```python
from build123d import *

# Parameters (mm, degrees)
CUT_EXTRUDE1_START = -20
CUT_EXTRUDE1_DEPTH = 20


with BuildPart() as part:
    # Sketch1 → Revolve1 (revolve)
    with BuildSketch(Plane.XY, mode=Mode.PRIVATE) as revolve1_sk:
        Polygon((0, 22.5), (4, 22.5), (4, -4), (10, -4), (10, -6), (0, -6), align=None)
    revolve(revolve1_sk.sketch.rotate(Axis((0, -6, 0), (0, 1, 0)), 90), axis=Axis((0, -6, 0), (0, 1, 0)))

    # Sketch2 → Cut-Extrude1 (cut)
    with BuildSketch(Plane(origin=(0, 22.5, 0), x_dir=(1, 0, 0), z_dir=(0, 1, 0)).offset(CUT_EXTRUDE1_START)):
        with BuildLine():
            Line((-2.645751311, -3), (2.645751311, -3))
            ThreePointArc((2.645751311, -3), (0, -4), (-2.645751311, -3))
        make_face()
    extrude(amount=CUT_EXTRUDE1_DEPTH, mode=Mode.SUBTRACT)


solid = part.part
```
Input: part model. Units: mm. Frame: model coordinates. A direction names the side the tool comes from. Give positions to 0.01 mm unless a question says otherwise; leave off trailing zeros. Write each loop counter-clockwise with the first axis right and the second up, starting at its lowest first coordinate (ties: lowest second). Pieces come first, ordered by that corner, then holes. Notation, with made-up numbers: (38.25, 52) - (91.25, 52) arc R27 cw to (91.25, 74) - close; hole circle Ø1 at (-40, 19). An arc over 180 degrees is marked (long way). Write item = value, one per line. Start each with the question number.
1) Cut plane C-C (y = 12). Return loops of the section in (x, z).
2) Material intervals for L1, parallel to Y at x = 7, z = -3.25; L2, parallel to Z at x = 3, y = 7.5; L3, parallel to X at y = 4.75, z = 2.25, sorted ascending. Write a range as [from, to].
3) Cut plane D-D (x = -3). Return loops of the section in (y, z), and give its area (3 significant figures).
4) Cut plane A-A (z = 0). Return loops of the section in (x, y), and give its area (3 significant figures).
5) Pin query (flat end, axial travel): pin 1 (6 mm diameter, centred on x = 5, y = -1.5, fed in from -Z); pin 2 (10 mm diameter, centred on y = 15.5, z = -0.5, fed in from +X); pin 3 (1.5 mm diameter, centred on x = -2, y = 1, fed in from +Z). Return the tip coordinate at first contact, or that it passes through.
6) Cut plane B-B (x = 0). Return loops of the section in (y, z).
7) Reachability of faces 1 (the face through (-0.1, -4, 4.3)), 2 (the face through (0, 2.5, 3.4)), 3 (the face through (0, 22.5, -1)) from +Z, -Z, +X, -X, +Y, -Y: full face, straight path, thin tool, end or side. Return the list, or none.
Answers follow:
q1.outline = (-2.65, 3) arc R4 ccw (long way) to (2.65, 3) - close
q2.L1 = [-6, -4]
q2.L2 = [-2.65, 2.65]
q2.L3 = [-3.31, 3.31]
q3.outline = (-6, -9.54) - (-4, -9.54) - (-4, -2.65) - (22.5, -2.65) - (22.5, 2.65) - (-4, 2.65) - (-4, 9.54) - (-6, 9.54) - close
q3.area = 178 mm^2
q4.outline = (-10, -6) - (10, -6) - (10, -4) - (4, -4) - (4, 22.5) - (-4, 22.5) - (-4, -4) - (-10, -4) - close
q4.area = 252 mm^2
q5.pin_1 = -9.43
q5.pin_2 = 4
q5.pin_3 = 3.8
q6.outline = (-6, -10) - (-4, -10) - (-4, -4) - (22.5, -4) - (22.5, 3) - (2.5, 3) - (2.5, 4) - (-4, 4) - (-4, 10) - (-6, 10) - close
q7.face_1 = +Y
q7.face_2 = +Z, +X, -X, +Y
q7.face_3 = +Z, -Z, +X, -X, +Y
